Autodesk Inventor part; units mm, degrees
ref_plane "YZ Plane" through (0, 0, 0) normal (1, 0, 0) x (0, 1, 0)
ref_plane "XZ Plane" through (0, 0, 0) normal (0, 1, 0) x (-1, 0, 0)
ref_plane "XY Plane" through (0, 0, 0) normal (0, 0, 1) x (1, 0, 0)
sketch "Sketch1" plane through (0, 0, 0) normal (0, 0, 1) x (1, 0, 0)
  line L0 (200, 0) -> (171.6283, 0) construction
  line L1 (200, 6) -> (200, 0)
  line L2 (171.6283, 6) -> (200, 6)
  line L3 (171.6283, 6) -> (171.6283, 0)
  line L4 (136.6283, 6) -> (136.6283, 0)
  line L5 (136.6283, 0) -> (171.6283, 0)
  line L6 (171.6283, 0) -> (171.6283, 6)
  line L7 (136.6283, 6) -> (171.6283, 6)
  line L8 (136.6283, 0) -> (117.5, 0) construction
  line L9 (136.6283, 6) -> (136.6283, 0)
  line L10 (117.5, 6) -> (136.6283, 6)
  line L11 (117.5, 6) -> (117.5, 0)
  line L12 (117.5, 0) -> (117.5, 6)
  line L13 (82.5, 6) -> (117.5, 6)
  line L14 (82.5, 6) -> (82.5, 0)
  line L15 (82.5, 0) -> (117.5, 0)
  line L16 (82.5, 0) -> (58.75, 0) construction
  line L17 (82.5, 6) -> (82.5, 0)
  line L18 (58.75, 6) -> (82.5, 6)
  line L19 (58.75, 6) -> (58.75, 0)
  line L20 (23.75, 6) -> (23.75, 0)
  line L21 (23.75, 0) -> (58.75, 0)
  line L22 (58.75, 0) -> (58.75, 6)
  line L23 (23.75, 6) -> (58.75, 6)
  line L24 (23.75, 0) -> (0, 0) construction
  line L25 (23.75, 6) -> (23.75, 0)
  line L26 (0, 6) -> (23.75, 6)
  line L27 (0, 0) -> (0, 6)
  line L28 (200, 6) -> (1.5061, 6)
  line L29 (1.5061, 6) -> (1.5061, -19)
  line L30 (1.5061, -19) -> (200, -19)
  line L31 (200, -19) -> (200, 6)
extrude "Extrusion1" add sketch "Sketch1" against normal blind 6 contours L1 L31 L30 L29 L26 L20 L21 L19 L18 L14 L15 L11 L10 L4 L5 L3 L2
sketch "Sketch2" plane through (0, 0, 0) normal (0, 0, 1) x (1, 0, 0)
  line L0 (200, 6) -> (171.6283, 6)
  line L1 (171.6283, 0) -> (171.6283, 6)
  line L2 (136.6283, 0) -> (171.6283, 0)
  line L3 (136.6283, 6) -> (136.6283, 0)
  line L4 (136.6283, 6) -> (117.5, 6)
  line L5 (117.5, 0) -> (82.5, 0)
  line L6 (82.5, 6) -> (82.5, 0)
  line L7 (82.5, 6) -> (58.75, 6)
  line L8 (58.75, 0) -> (58.75, 6)
  line L9 (58.75, 0) -> (23.75, 0)
  line L10 (23.75, 0) -> (23.75, 6)
  line L11 (23.75, 6) -> (1.5061, 6)
  line L12 (1.5061, -19) -> (200, -19) construction
  line L13 (200, -19) -> (1.5061, -19) construction
  line L14 (195.1496, -19) -> (195.1496, 6) construction
  line L15 (171.6283, 6) -> (200, 6) construction
  line L16 (195.1496, -6.5) -> (183.8978, -6.5) construction
  line L17 (200, -19) -> (171.6283, -19)
  line L18 (171.6283, -13) -> (171.6283, -19)
  line L19 (136.6283, -13) -> (171.6283, -13)
  line L20 (136.6283, -19) -> (136.6283, -13)
  line L21 (136.6283, -19) -> (117.5, -19)
  line L22 (117.5, -13) -> (82.5, -13)
  line L23 (82.5, -19) -> (82.5, -13)
  line L24 (82.5, -19) -> (58.75, -19)
  line L25 (58.75, -13) -> (58.75, -19)
  line L26 (58.75, -13) -> (23.75, -13)
  line L27 (23.75, -13) -> (23.75, -19)
  line L28 (23.75, -19) -> (1.5061, -19)
  line L29 (195.1496, 6) -> (195.1496, -19) construction
  line L30 (171.6283, -19) -> (200, -19) construction
  line L31 (117.5, -13) -> (117.5, -19)
  line L32 (82.5, -19) -> (117.5, -19)
  line L33 (23.75, -19) -> (58.75, -19)
  line L34 (171.6283, -19) -> (136.6283, -19)
  point P0 (0, 0)
  point P1 (0, -13)
extrude "Extrusion2" cut sketch "Sketch2" against normal through all
move faces "Move1" translate (-1.5061, 0, 0) faces at (1.5061, -2.3333, -2)
properties part number "top"
Build history of the part. All positions in model axes, mm. A direction names the side the tool comes from. Give positions to 0.01 mm unless a question says otherwise; leave off trailing zeros. Loops run counter-clockwise (first coordinate to the right, second up) from the corner with the lowest first, then second, coordinate; pieces in that order, holes last.
Item 1: Flat gauge pin, fed straight in: pin 1 (3 mm diameter, centred on x = 146.5, z = -2.5, fed in from +Y). Where does the tip first touch, or does it go through?
Answers follow:
pin 1: stops at y = 0
Item 2: Slice it at C-C, the plane x = 53.5. List the corners of the cut face in (y, z), and give its area (3 significant figures).
Answers follow:
outline: (-13, -6) - (0, -6) - (0, 0) - (-13, 0) - close
area: 78.0 mm2
Item 3: Drill centre lines: line 1 (X direction, y = -15.75, z = -0.45); line 2 (Y direction, x = 85, z = -3.5). Where is each one in solid material? Low to high.
Answers follow:
line 1: x = 0 to 23.75, 58.75 to 82.5, 117.5 to 136.63, 171.63 to 200
line 2: y = -13 to 0
Item 4: Slice it at B-B, the plane z = -1.8. List the corners of the cut face in (x, y).
Answers follow:
outline: (0, -19) - (23.75, -19) - (23.75, -13) - (58.75, -13) - (58.75, -19) - (82.5, -19) - (82.5, -13) - (117.5, -13) - (117.5, -19) - (136.63, -19) - (136.63, -13) - (171.63, -13) - (171.63, -19) - (200, -19) - (200, 6) - (171.63, 6) - (171.63, 0) - (136.63, 0) - (136.63, 6) - (117.5, 6) - (117.5, 0) - (82.5, 0) - (82.5, 6) - (58.75, 6) - (58.75, 0) - (23.75, 0) - (23.75, 6) - (0, 6) - close
Item 5: Pull direction X, two halves, no side cores. Call faces 4 (the face through (200, -6, -3)), 5 (the face through (23.75, -16, -3)), 6 (the face through (70, 6, -3)): released by +X, released by -X, zero draft, split by the parting line, or undercut.
Answers follow:
face 4: released by +X
face 5: undercut
face 6: zero draft
Item 6: Which spindle directions (+Z, -Z, +X, -X, +Y, -Y) get a long thin tool onto all of the face, cutting with end or side? Do faces 1 (the face through (100, -13, -3)), 2 (the face through (136.628, 3, -3)), 3 (the face through (127, 6, -3)). Say none if no direction does.
Answers follow:
face 1: +Z, -Z, -Y
face 2: +Z, -Z, +Y
face 3: +Z, -Z, +X, -X, +Y
Item 7: Slice it at A-A, the plane y = -15.5. List the corners of the cut face in (x, z).
Answers follow:
outline: (0, -6) - (23.75, -6) - (23.75, 0) - (0, 0) - close; (58.75, -6) - (82.5, -6) - (82.5, 0) - (58.75, 0) - close; (117.5, -6) - (136.63, -6) - (136.63, 0) - (117.5, 0) - close; (171.63, -6) - (200, -6) - (200, 0) - (171.63, 0) - close
